from build123d import *

# Parameters (mm, degrees)
F0_R     = 30
F1_DEPTH = 35
F3_T     = -27.5
F4_W     = 14
F4_H     = 38
F5_DEPTH = 10
F6_R     = 2.5
F7_DEPTH = 5


with BuildPart() as f1:
    # F0 (on Front) → F1 (new body)
    with BuildSketch(Plane.XZ):
        Circle(F0_R)
    extrude(amount=F1_DEPTH)

    # F3
    f3_openings = [f1.faces().sort_by_distance(p)[0] for p in [
        (0, 0, 0),
    ]]
    offset(amount=F3_T, openings=f3_openings)

    # F4 (on face) → F5 (cut)
    with BuildSketch(Plane.XZ.offset(35)):
        with Locations((-12.541194, 0.233546)):
            Rectangle(F4_W, F4_H)
        with Locations((11.464599, 0.298456)):
            Rectangle(F4_W, F4_H)
    extrude(amount=-F5_DEPTH, mode=Mode.SUBTRACT)

    # F6 (on face) → F7 (cut)
    with BuildSketch(Plane.XZ.offset(35)):
        Circle(F6_R)
        with Locations((-24, 0)):
            Circle(F6_R)
        with Locations((24, 0)):
            Circle(F6_R)
    extrude(amount=-F7_DEPTH, mode=Mode.SUBTRACT)


solid = f1.part
The listing builds one solid part. Answer for the finished solid, in the listing's coordinates (mm). A direction names the side the tool comes from. Round coordinates to 2 decimals unless told otherwise and drop trailing zeros. Write each loop counter-clockwise with the first axis right and the second up, starting at its lowest first coordinate (ties: lowest second). Pieces come first, ordered by that corner, then holes. Notation, with made-up numbers: (14, -28) - (45, -28) arc R15 ccw to (45, -11) - close; hole circle Ø5 at (-0.5, -30.75). An arc over 180 degrees is marked (long way). Use one line per item in the form item = value. Start each with the question number.
Item 1: A cutting plane is placed at C-C (z = 0). Write down the section's boundary in (x, y).
Item 2: A cutting plane is placed at B-B (y = -26.5). Write down the section's boundary in (x, z), plus the area to 3 significant figures.
Item 3: Find the intervals of material crossed by line 1 (Z direction, x = 0, y = -3); line 2 (X direction, y = -28.5, z = -6); line 3 (X direction, y = -29, z = -3), in increasing order. Write a range as [from, to].
Item 4: A cutting plane is placed at A-A (y = -32.5). Write down the section's boundary in (x, z).
Item 5: Flat-ended cylindrical pins translate along their axes: pin 1 Ø4 at (x, y) = (6.5, -20.5) entering from -Z; pin 2 Ø4 at (x, z) = (0, 0) entering from +Y; pin 3 Ø1 at (x, y) = (-12.5, -26) entering from +Z; pin 4 Ø1 at (x, z) = (-21.5, 15) entering from +Y. Find the tip coordinate at first contact, or state that the pin passes through.
Item 6: Determine the mould class of faces 1 (the flat face through (-24, -30, 0)), 2 (the flat face through (6, 0, 0)), 3 (the cylindrical face through (-29.97, -17.26, 1.32)) for opening direction X: +X half, -X half, draft (parallel to the pull), parting line (faces both ways), or undercut.
Item 7: A tool of negligible diameter and unlimited length cuts with its end or side. For faces 4 (the flat face through (0, -7.5, 0)), 5 (the flat face through (0, -35, -6)), 6 (the cylindrical face through (-0.54, -32.53, -2.44)), from which of +Z, -Z, +X, -X, +Y, -Y can it reach the whole face along a straight path? Write none if from no direction.
Item 8: A cutting plane is placed at D-D (x = 24). Write down the section's boundary in (y, z), plus the area to 4 significant figures.
The answers:
q1.outline = (-30, -35) - (-26.5, -35) - (-26.5, -30) - (-21.5, -30) - (-21.5, -35) - (-19.54, -35) - (-19.54, -25) - (-5.54, -25) - (-5.54, -35) - (-2.5, -35) - (-2.5, -30) - (2.5, -30) - (2.5, -35) - (4.46, -35) - (4.46, -25) - (18.46, -25) - (18.46, -35) - (21.5, -35) - (21.5, -30) - (26.5, -30) - (26.5, -35) - (30, -35) - (30, 0) - (2.5, 0) - (2.5, -7.5) - (-2.5, -7.5) - (-2.5, 0) - (-30, 0) - close
q2.outline = circle Ø60 at (0, 0); hole (-19.54, -18.77) - (-5.54, -18.77) - (-5.54, 19.23) - (-19.54, 19.23) - close; hole (4.46, -18.7) - (18.46, -18.7) - (18.46, 19.3) - (4.46, 19.3) - close
q2.area = 1,760 mm^2
q3.line_1 = [-30, -2.5], [2.5, 30]
q3.line_2 = [-29.39, -19.54], [-5.54, 4.46], [18.46, 29.39]
q3.line_3 = [-29.85, -19.54], [-5.54, 4.46], [18.46, 29.85]
q4.outline = circle Ø60 at (0, 0); hole circle Ø5 at (-24, 0); hole (-19.54, -18.77) - (-5.54, -18.77) - (-5.54, 19.23) - (-19.54, 19.23) - close; hole circle Ø5 at (0, 0); hole (4.46, -18.7) - (18.46, -18.7) - (18.46, 19.3) - (4.46, 19.3) - close; hole circle Ø5 at (24, 0)
q5.pin_1 = -29.66
q5.pin_2 = -7.5
q5.pin_3 = 27.5
q5.pin_4 = 0
q6.face_1 = undercut
q6.face_2 = draft
q6.face_3 = parting line
q7.face_4 = +Y
q7.face_5 = +Z, -Z, +X, -X, -Y
q7.face_6 = -Y
q8.outline = (-35, -18) - (0, -18) - (0, 18) - (-35, 18) - (-35, 2.5) - (-30, 2.5) - (-30, -2.5) - (-35, -2.5) - close
q8.area = 1,235 mm^2
